Could you check a few things on this model? Use its own coordinates, in mm. A direction names the side the tool comes from. Give positions to 0.01 mm unless a question says otherwise; leave off trailing zeros. Order: outer loops, then holes, each group sorted by start corner. A loop starts at its lowest first (then second) coordinate and runs counter-clockwise, first axis right, second up.
from build123d import *

# Parameters (mm, degrees)
BLANKSKE_W              = 152.4
BLANKSKE_H              = 28.575
BLANK_DEPTH             = 11.811
TOOTHCUTSIM_DEPTH       = 156.504952802
TEETHCUTS_COUNT         = 16
TEETHCUTS_PITCH         = 9.974556664
SKETCH2_W               = 23.941257987
SKETCH2_H               = 28.575
BOSS_EXTRUDE1_DEPTH     = 11.811
CUT_EXTRUDE1_DEPTH      = 156.504952802
CUT_EXTRUDE1_DEPTH_BACK = 156.504952802
CUT_EXTRUDE5_DEPTH      = 156.504952802
CUT_EXTRUDE5_DEPTH_BACK = 156.504952802
SKETCH5_R               = 2.413
CUT_EXTRUDE6_DEPTH      = 12.446


with BuildPart() as part:
    # BlankSke → Blank (new body)
    with BuildSketch(Plane.XY):
        with Locations((76.2, 14.2875)):
            Rectangle(BLANKSKE_W, BLANKSKE_H)
    extrude(amount=-BLANK_DEPTH)

    # TooCutSkeSim → ToothCutSim (cut, through all)
    with BuildSketch(Plane.XY):
        Polygon((1.392032299, 21.43125), (-1.392032299, 21.43125), (-4.001389504, 28.6004), (4.001389504, 28.6004), align=None)
    toothcutsim = extrude(amount=-TOOTHCUTSIM_DEPTH, mode=Mode.SUBTRACT)

    # TeethCuts: ToothCutSim ×16
    with Locations(*[(i * TEETHCUTS_PITCH, 0, 0) for i in range(1, TEETHCUTS_COUNT)]):
        add(toothcutsim, mode=Mode.SUBTRACT)

    # Sketch2 → Boss-Extrude1 (add)
    with BuildSketch(Plane.XY):
        with Locations((11.970628994, 14.2875)):
            Rectangle(SKETCH2_W, SKETCH2_H)
    extrude(amount=-BOSS_EXTRUDE1_DEPTH)

    # Sketch3 → Cut-Extrude1 (cut, two sides)
    with BuildSketch(Plane.XY) as cut_extrude1_sk:
        Polygon((-316.449184205, 12.7), (0, 12.7), (25.4, 12.7), (25.4, 15.875), (0, 15.875), (-316.449184205, 15.875), (-949.347552615, 15.875), (-949.347552615, 12.7), align=None)
    extrude(amount=CUT_EXTRUDE1_DEPTH, mode=Mode.SUBTRACT)
    extrude(cut_extrude1_sk.sketch, amount=-CUT_EXTRUDE1_DEPTH_BACK, mode=Mode.SUBTRACT)

    # Sketch4 → Cut-Extrude5 (cut, two sides)
    with BuildSketch(Plane(origin=(0, 28.575, 0), x_dir=(1, 0, 0), z_dir=(0, 1, 0))) as cut_extrude5_sk:
        Polygon((-315.09434574, 6.69925), (0, 6.69925), (25.4, 6.69925), (25.4, 5.11175), (0, 5.11175), (-315.09434574, 5.11175), (-945.283037219, 5.11175), (-945.283037219, 6.69925), align=None)
    extrude(amount=CUT_EXTRUDE5_DEPTH, mode=Mode.SUBTRACT)
    extrude(cut_extrude5_sk.sketch, amount=-CUT_EXTRUDE5_DEPTH_BACK, mode=Mode.SUBTRACT)

    # Sketch5 → Cut-Extrude6 (cut)
    with BuildSketch(Plane.XY):
        with Locations(Location((6.35, 22.225, 0), (0, 0, 180))):
            Circle(SKETCH5_R)
        with Locations(Location((19.05, 22.225, 0), (0, 0, 180))):
            Circle(SKETCH5_R)
        with Locations((19.05, 6.35)):
            Circle(SKETCH5_R)
        with Locations((6.35, 6.35)):
            Circle(SKETCH5_R)
    extrude(amount=-CUT_EXTRUDE6_DEPTH, mode=Mode.SUBTRACT)


solid = part.part
Item 1: Imagine slicing it at B-B on y = 6.35. List the corners of the cut face in (x, z) for me, then the cut area to 3 significant figures.
Findings:
outline: (0, -11.81) - (3.94, -11.81) - (3.94, -6.7) - (0, -6.7) - close; (0, -5.11) - (3.94, -5.11) - (3.94, 0) - (0, 0) - close; (8.76, -11.81) - (16.64, -11.81) - (16.64, -6.7) - (8.76, -6.7) - close; (8.76, -5.11) - (16.64, -5.11) - (16.64, 0) - (8.76, 0) - close; (21.46, -11.81) - (152.4, -11.81) - (152.4, 0) - (21.46, 0) - (21.46, -5.11) - (25.4, -5.11) - (25.4, -6.7) - (21.46, -6.7) - close
area: 1,660 mm2
Item 2: Imagine slicing it at A-A on x = 13. List the corners of the cut face in (y, z) for me (3 decimals), then the cut area to 3 significant figures.
Findings:
outline: (0, -11.811) - (12.7, -11.811) - (12.7, -6.699) - (0, -6.699) - close; (0, -5.112) - (12.7, -5.112) - (12.7, 0) - (0, 0) - close; (15.875, -11.811) - (28.575, -11.811) - (28.575, -6.699) - (15.875, -6.699) - close; (15.875, -5.112) - (28.575, -5.112) - (28.575, 0) - (15.875, 0) - close
area: 260 mm2
Item 3: Imagine slicing it at C-C on z = -10.5. Give the number of separate pieces and of enclosed holes in the cut face, then the cut area to 3 significant figures.
Findings:
separate pieces: 1
enclosed holes: 4
area: 3,700 mm2
Item 4: For faces 4 (the cylindrical face through (16.64, 6.46, -2.52)), 5 (the flat face through (13, 15.875, -9)), 6 (the flat face through (50, 21.431, -6)), which set-ups out of +Z, -Z, +X, -X, +Y, -Y let a thin tool reach every point of the face, with its end or its side?
Findings:
face 4: +Z, -Z
face 5: +Z, -Z, -X
face 6: +Z, -Z, +Y
Item 5: We'd pull the mould along X, two halves only. Please class faces 1 (the flat face through (0, 22, -9)), 2 (the flat face through (13, 12.7, -3)), 3 (the flat face through (52.6, 25.1, -5.8)): +X half, -X half, draft (parallel to the pull), parting line (faces both ways), or undercut.
Findings:
face 1: -X half
face 2: draft
face 3: undercut
Item 6: Please list where these lines run through material, in increasing order: line 1 along Y through (x, z) = (6.35, -4) (3 decimals); line 2 along X through (y, z) = (6.5, -10); line 3 along Z through (x, y) = (22, 20.75).
Findings:
line 1: y = 0 to 3.937, 8.763 to 12.7, 15.875 to 19.812, 24.638 to 28.575
line 2: x = 0 to 3.94, 8.76 to 16.64, 21.46 to 152.4
line 3: z = -11.81 to -6.7, -5.11 to 0
Item 7: For pin 1 (2 mm diameter, centred on x = 99.5, z = -6, fed in from +Y); pin 2 (4.5 mm diameter, centred on x = 6.35, y = 22.225, fed in from -Z), each with a flat end and sliding along its axis, tell me the tip position at first contact or that it passes through.
Findings:
pin 1: stops at y = 21.43
pin 2: passes through
Item 8: Imagine slicing it at D-D on x = 82.5. List the corners of the cut face in (y, z) for me.
Findings:
outline: (0, -11.81) - (25.03, -11.81) - (25.03, 0) - (0, 0) - close
